Part model, mm, in its own coordinate system. A direction names the side the tool comes from. Give positions to 0.01 mm unless a question says otherwise; leave off trailing zeros. Order: outer loops, then holes, each group sorted by start corner. A loop starts at its lowest first (then second) coordinate and runs counter-clockwise, first axis right, second up. Notation, with made-up numbers: (28, 54.25) -> (44, 54.25) arc R20 ccw to (44, 83.25) -> close; hole circle Ø9 at (54.25, -27). An arc over 180 degrees is marked (long way). Write item = value, one per line. Start each with the question number.
(1) Saw through at A-A, the plane y = 102.5. List the corners of the cut face in (x, z), then the cut area to 4 significant figures.
(2) Which spindle directions (+Z, -Z, +X, -X, +Y, -Y) get a long thin tool onto all of the face, cutting with end or side? Do faces 1 (the flat face through (-41.631, 99, 12)), 2 (the flat face through (229, 182, 0)). Say none if no direction does.
(3) Flat gauge pin, fed straight in: pin 1 (10 mm diameter, centred on x = 211, y = 209, fed in from -Z). Where does the tip first touch, or does it go through?
(4) Probe line 1 along X through (y, z) = (124.5, 2.25). List the from-to ranges inside material, lowest first. Write a range as from..to.
(5) Two-plate mould, pull along Y, no slides. Class faces 3 (the flat face through (229, -41.41, 12)), 4 (the flat face through (238, 398.59, 12)), 5 (the flat face through (528.449, 99, 12)), 6 (the flat face through (229, 182, 25)): pulls with the +Y half, pulls with the -Y half, needs draft (parallel to the pull), parting line crosses it, or undercut.
from build123d import *

# Parameters (mm, degrees)
F0_R     = 2.0293084654
F0_R_2   = 2.7851350605
F1_DEPTH = 25


with BuildPart() as f1:
    # F0 (on Top) → F1 (new body)
    with BuildSketch(Plane.XY):
        Polygon((-38.5909078717, 398.5895687342), (-71.5909078717, 398.5895687342), (-71.5909078717, -41.4104312658), (-38.5909078717, -41.4104312658), (-38.5909078717, 191.306501627), align=None)
        with Locations((-59.2456907034, -27.969462797)):
            Circle(F0_R, mode=Mode.SUBTRACT)
        with BuildLine():
            ThreePointArc((-56.6312761605, 58.5325606167), (-60.1668100664, 59.9970267108), (-61.6312761605, 63.5325606167))
            Line((-61.6312761605, 63.5325606167), (-61.6312761605, 133.5325606167))
            ThreePointArc((-61.6312761605, 133.5325606167), (-60.1668100664, 137.0680945227), (-56.6312761605, 138.5325606167))
            Line((-56.6312761605, 138.5325606167), (-41.6312761605, 138.5325606167))
            Line((-41.6312761605, 138.5325606167), (-41.6312761605, 58.5325606167))
            Line((-41.6312761605, 58.5325606167), (-56.6312761605, 58.5325606167))
        make_face(mode=Mode.SUBTRACT)
        with Locations((-56.7024089396, 384.5269083977)):
            Circle(F0_R_2, mode=Mode.SUBTRACT)
        Polygon((505.4090921283, 398.5895687342), (-38.5909078717, 398.5895687342), (-38.5909078717, 191.306501627), (-38.5909078717, -41.4104312658), (505.4090921283, -41.4104312658), (505.4090921283, 191.306501627), align=None)
        Polygon((538.4090921283, 398.5895687342), (505.4090921283, 398.5895687342), (505.4090921283, 191.306501627), (505.4090921283, -41.4104312658), (538.4090921283, -41.4104312658), align=None)
        with Locations((526.0638749599, -27.969462797)):
            Circle(F0_R, mode=Mode.SUBTRACT)
        with BuildLine():
            Line((508.449460417, 138.5325606167), (523.449460417, 138.5325606167))
            ThreePointArc((523.449460417, 138.5325606167), (526.984994323, 137.0680945227), (528.449460417, 133.5325606167))
            Line((528.449460417, 133.5325606167), (528.449460417, 63.5325606167))
            ThreePointArc((528.449460417, 63.5325606167), (526.984994323, 59.9970267108), (523.449460417, 58.5325606167))
            Line((523.449460417, 58.5325606167), (508.449460417, 58.5325606167))
            Line((508.449460417, 58.5325606167), (508.449460417, 138.5325606167))
        make_face(mode=Mode.SUBTRACT)
        with Locations((523.5205931962, 384.5269083977)):
            Circle(F0_R_2, mode=Mode.SUBTRACT)
    extrude(amount=F1_DEPTH)


solid = f1.part
Results list:
q1.outline = (-71.59, 0) -> (-61.63, 0) -> (-61.63, 25) -> (-71.59, 25) -> close; (-41.63, 0) -> (508.45, 0) -> (508.45, 25) -> (-41.63, 25) -> close; (528.45, 0) -> (538.41, 0) -> (538.41, 25) -> (528.45, 25) -> close
q1.area = 14,250 mm^2
q2.face_1 = +Z, -Z
q2.face_2 = -Z, +X, -X, +Y, -Y
q3.pin_1 = 0
q4.line_1 = -71.59..-61.63, -41.63..508.45, 528.45..538.41
q5.face_3 = pulls with the -Y half
q5.face_4 = pulls with the +Y half
q5.face_5 = undercut
q5.face_6 = needs draft
